Geometry check sheet. Reference: the model listing, model coordinates, mm. Face numbers are marked on the shaded views. Round coordinates to 2 decimals unless told otherwise and drop trailing zeros. Loops run counter-clockwise (first coordinate to the right, second up) from the corner with the lowest first, then second, coordinate; pieces in that order, holes last. Notation, with made-up numbers: M 83.25,-35.75 L 131.25,-35.75 A16 ccw 131.25,-24.75 Z; hole C 5.5,27 d3. An arc over 180 degrees is marked long. Answer in a Markdown table with one row per item. Add a question column.
Autodesk Fusion 360 part; units mm, degrees
sketch "Sketch1" plane through (0, 0, 0) normal (0, 0, 1) x (1, 0, 0)
  line L0 (0, 0) -> (20.3, 0)
  line L1 (20.3, 0) -> (20.3, 15.6)
  line L2 (20.3, 15.6) -> (0, 15.6)
  line L3 (0, 15.6) -> (0, 0)
  line L4 (9, 12.9) -> (12.3, 12.9)
  line L5 (12.3, 12.9) -> (12.3, 11.22)
  line L6 (12.3, 11.22) -> (9, 11.22)
  line L7 (9, 11.22) -> (9, 12.9)
  line L8 (0.7, 2.7) -> (19.6, 2.7)
  line L9 (19.6, 2.7) -> (19.6, 0.7)
  line L10 (19.6, 0.7) -> (0.7, 0.7)
  line L11 (0.7, 0.7) -> (0.7, 2.7)
  dimension "d1" = 20.3
  dimension "d2" = 15.6
  dimension "d3" = 3.3
  dimension "d4" = 1.68
  dimension "d5" = 2.7
  dimension "d6" = 8
  dimension "d7" = 0.7
  dimension "d8" = 2
  dimension "d9" = 0.7
  dimension "d10" = 0.7
extrude "Extrude1" add sketch "Sketch1" along normal blind 1.6 contours L0 L1 L2 L3 | L4 L5 L6 L7 | L8 L9 L10 L11
extrude "Extrude2" add sketch "Sketch1" along normal blind 3.6 contours L4 L5 L6 L7
extrude "Extrude3" add sketch "Sketch1" along normal blind 3.6 and the other way blind 0.5 contours L8 L9 L10 L11
sketch "Sketch2" plane through (0, 0, 1.6) normal (0, 0, 1) x (-1, 0, 0)
  line L0 (-0.7, -0.7) -> (-0.7, -2.7)
  line L1 (-0.7, -2.7) -> (-19.6, -2.7)
  line L2 (-19.6, -2.7) -> (-19.6, -0.7)
  line L3 (-19.6, -0.7) -> (-0.7, -0.7)
  line L4 (-9, -11.22) -> (-9, -12.9)
  line L5 (-9, -12.9) -> (-12.3, -12.9)
  line L6 (-12.3, -12.9) -> (-12.3, -11.22)
  line L7 (-12.3, -11.22) -> (-9, -11.22)
  line L8 (0, -15.6) -> (0, 0)
  line L9 (0, 0) -> (-20.3, 0)
  line L10 (-20.3, 0) -> (-20.3, -15.6)
  line L11 (-20.3, -15.6) -> (0, -15.6)
  circle A0 centre (-2.2, -13.2) radius 1.5
  line L12 (-20.3, -15.6) -> (0, -15.6)
  line L13 (0, -15.6) -> (0, 0)
  line L14 (-10.15, -15.6) -> (-10.15, -9.9904) construction
  circle A1 centre (-18.1, -13.2) radius 1.5
  dimension "d19" = 3
  dimension "d21" = 2.4
  dimension "d22" = 2.2
extrude "Extrude4" cut sketch "Sketch2" against normal through all contours A0 | A1
equation "d21 = 0.9 mm + ( d19 / 2 )"
equation "d22 = 0.7 mm + ( d19 / 2 )"
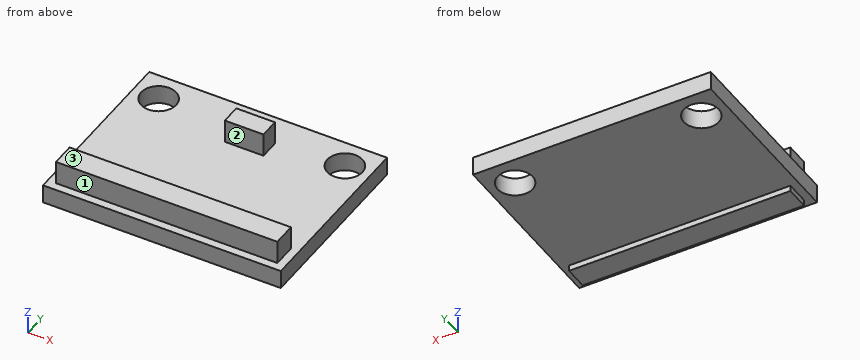
1) Draft check along Y on the marked faces 1, 2 and 3. Enter one of: +Y half, -Y half, draft (parallel to the pull), parting line (faces both ways), or undercut.
2) Cross-section at B-B, the plane x = 18.1. Record the boundary of the cut face in (y, z), plus the area to 3 significant figures.
3) Go/stop test with flat-tipped pins: pin 1 (3.5 mm diameter, centred on x = 18.1, y = 13.2, fed in from -Z); pin 2 (0.6 mm diameter, centred on y = 1, z = -0.5, fed in from -X); pin 3 (1.6 mm diameter, centred on x = 10, z = 3, fed in from +Y). Record where each tip stops, or that it passes through.
4) Cross-section at D-D, the plane z = 0.65. Record the boundary of the cut face in (x, y), plus the area to 3 significant figures.
5) Cross-section at A-A, the plane y = 13.2. Record the boundary of the cut face in (x, z).
6) Cross-section at C-C, the plane x = 15. Record the boundary of the cut face in (y, z), plus the area to 3 significant figures.
7) Thickness scan on L1, parallel to X at y = 13.2, z = 0.3; L2, parallel to Y at x = 18.1, z = 0.85; L3, parallel to X at y = 12.5, z = 1.35. Record the ranges inside material, lowest first. Write a range as [from, to].
Worked answers:
| question | item | result |
|---|---|---|
| 1 | face 1 | -Y half |
| 1 | face 2 | undercut |
| 1 | face 3 | draft |
| 2 | outline | M 0,0 L 0.7,0 L 0.7,-0.5 L 2.7,-0.5 L 2.7,0 L 11.7,0 L 11.7,1.6 L 2.7,1.6 L 2.7,3.6 L 0.7,3.6 L 0.7,1.6 L 0,1.6 Z; M 14.7,0 L 15.6,0 L 15.6,1.6 L 14.7,1.6 Z |
| 2 | area | 25.2 mm2 |
| 3 | pin 1 | stops at z = 0 |
| 3 | pin 2 | stops at x = 0.7 |
| 3 | pin 3 | stops at y = 12.9 |
| 4 | outline | M 0,0 L 20.3,0 L 20.3,15.6 L 0,15.6 Z; hole C 2.2,13.2 d3; hole C 18.1,13.2 d3 |
| 4 | area | 303 mm2 |
| 5 | outline | M 0,0 L 0.7,0 L 0.7,1.6 L 0,1.6 Z; M 3.7,0 L 16.6,0 L 16.6,1.6 L 3.7,1.6 Z; M 19.6,0 L 20.3,0 L 20.3,1.6 L 19.6,1.6 Z |
| 6 | outline | M 0,0 L 0.7,0 L 0.7,-0.5 L 2.7,-0.5 L 2.7,0 L 15.6,0 L 15.6,1.6 L 2.7,1.6 L 2.7,3.6 L 0.7,3.6 L 0.7,1.6 L 0,1.6 Z |
| 6 | area | 30.0 mm2 |
| 7 | L1 | x = [0, 0.7], [3.7, 16.6], [19.6, 20.3] |
| 7 | L2 | y = [0, 11.7], [14.7, 15.6] |
| 7 | L3 | x = [0, 0.87], [3.53, 16.77], [19.43, 20.3] |
